```python
from build123d import *

# Parameters (mm, degrees)
SKETCH_1_R               = 51.220940725
EXTRUDE_1_DEPTH          = 2
SKETCH_2_R               = 3.5
EXTRUDE_2_DEPTH          = 5
PATTERN_CIRCULAR_1_COUNT = 6
SKETCH_3_R               = 2.5
CUT_EXTRUDE_1_DEPTH      = 3
PATTERN_CIRCULAR_2_COUNT = 6
SKETCH_4_R               = 2.5
EXTRUDE_3_DEPTH          = 11
SKETCH_5_R               = 3.5
EXTRUDE_4_DEPTH          = 7
SKETCH_6_R               = 5
EXTRUDE_5_DEPTH          = 20
SKETCH_7_R               = 6
EXTRUDE_6_DEPTH          = 5
SKETCH_8_R               = 2.5
CUT_EXTRUDE_2_DEPTH      = 7


with BuildPart() as part:
    # 草图1 → 凸台-拉伸1 (new body)
    with BuildSketch(Plane(origin=(0, 0, 0), x_dir=(0, 0, -1), z_dir=(1, 0, 0))):
        Circle(SKETCH_1_R)
    extrude(amount=EXTRUDE_1_DEPTH)

    # 草图2 → 凸台-拉伸2 (add)
    with BuildSketch(Plane(origin=(2, 0, 0), x_dir=(0, 0, -1), z_dir=(1, 0, 0))):
        with Locations((0, 45)):
            Circle(SKETCH_2_R)
    extrude_2 = extrude(amount=EXTRUDE_2_DEPTH)

    # 阵列(圆周)1: 凸台-拉伸2 ×6 about axis
    pattern_circular_1_axis = Axis((0, 0, 0), (1, 0, 0))
    for i in range(1, PATTERN_CIRCULAR_1_COUNT):
        add(extrude_2.rotate(pattern_circular_1_axis, i * 360 / PATTERN_CIRCULAR_1_COUNT))

    # 草图3 → 切除-拉伸1 (cut)
    with BuildSketch(Plane(origin=(7, 0, 0), x_dir=(0, 0, -1), z_dir=(1, 0, 0))):
        with Locations((0, 45)):
            Circle(SKETCH_3_R)
    cut_extrude_1 = extrude(amount=-CUT_EXTRUDE_1_DEPTH, mode=Mode.SUBTRACT)

    # 阵列(圆周)2: 切除-拉伸1 ×6 about axis
    pattern_circular_2_axis = Axis((0, 0, 0), (1, 0, 0))
    for i in range(1, PATTERN_CIRCULAR_2_COUNT):
        add(cut_extrude_1.rotate(pattern_circular_2_axis, i * 360 / PATTERN_CIRCULAR_2_COUNT), mode=Mode.SUBTRACT)

    # 草图4 → 凸台-拉伸3 (add)
    with BuildSketch(Plane(origin=(2, 0, 0), x_dir=(0, 0, -1), z_dir=(1, 0, 0))):
        Circle(SKETCH_4_R)
    extrude(amount=EXTRUDE_3_DEPTH)

    # 草图5 → 凸台-拉伸4 (add)
    with BuildSketch(Plane(origin=(2, 0, 0), x_dir=(0, 0, -1), z_dir=(1, 0, 0))):
        Circle(SKETCH_5_R)
    extrude(amount=EXTRUDE_4_DEPTH)

    # 草图6 → 凸台-拉伸5 (add)
    with BuildSketch(Plane.ZY):
        with Locations(Location((0, 0, 0), (0, 0, 180))):
            Circle(SKETCH_6_R)
    extrude(amount=EXTRUDE_5_DEPTH)

    # 草图7 → 凸台-拉伸6 (add)
    with BuildSketch(Plane.ZY):
        with Locations(Location((0, 0, 0), (0, 0, 180))):
            Circle(SKETCH_7_R)
    extrude(amount=EXTRUDE_6_DEPTH)

    # 草图8 → 切除-拉伸2 (cut)
    with BuildSketch(Plane.ZY.offset(20)):
        with Locations(Location((0, 0, 0), (0, 0, 180))):
            Circle(SKETCH_8_R)
    extrude(amount=-CUT_EXTRUDE_2_DEPTH, mode=Mode.SUBTRACT)


solid = part.part
```
For this review, take the finished solid that the model builds, in its own axes (mm). A direction names the side the tool comes from. Round coordinates to 2 decimals unless told otherwise and drop trailing zeros. Write each loop counter-clockwise with the first axis right and the second up, starting at its lowest first coordinate (ties: lowest second). Pieces come first, ordered by that corner, then holes. Notation, with made-up numbers: (48, -34) - (60, -34) arc R20 cw to (60, -17) - close; hole circle Ø4 at (1.5, 60.5). An arc over 180 degrees is marked (long way). Answer as CSV lines item,"result". Start each with the question number.
(1) Add section C-C, the plane z = 9. State the section outline as (x, y) points, plus the area to 3 significant figures.
(2) Add section D-D, the plane y = 45. State the section outline as (x, z) points, plus the area to 3 significant figures.
(3) Add section B-B, the plane x = 5.5. State how many separate pieces and enclosed holes the cut face has, plus the area to 3 significant figures.
(4) For pin 1 (1.5 mm diameter, centred on y = 23, z = -38, fed in from +X); pin 2 (5 mm diameter, centred on y = -34, z = 34, fed in from -X); pin 3 (8 mm diameter, centred on y = -22.5, z = 38.97, fed in from +X), all flat-tipped, find the tip position at first contact; note any pin that passes through.
(5) Machinability: for faces 5 (the flat face through (7, -23, -36)), 6 (the flat face through (4, -23, 39)), 7 (the cylindrical face through (-16.5, -0.1, 2.5)), which of the approach directions +Z, -Z, +X, -X, +Y, -Y give a long, thin tool a straight path to every point of the face, cutting with its end or side? Answer none if there is none.
(6) For line 1 (X direction, y = -17, z = -23.5); line 2 (X direction, y = 23.5, z = 37.5); line 3 (Y direction, x = 1.5, z = 19), list the stretches that pass through material, from the lowest coordinate up.
(7) Mouldability with a two-part tool opening along Y and no side actions: class faces 1 (the flat face through (-5, -4, 4)), 2 (the cylindrical face through (10.97, -2.44, 0.54)), 3 (the cylindrical face through (5.521, -22.39, -36.474)), 4 (the cylindrical face through (4.465, 20.135, -41.551)) as +Y half, -Y half, draft (parallel to the pull), parting line (faces both ways), or undercut.
(8) Add section A-A, the plane y = 0. State the section outline as (x, z) points, plus the area to 3 significant figures.
From the geometry:
1,outline,"(0, -50.42) - (2, -50.42) - (2, 50.42) - (0, 50.42) - close"
1,area,"202 mm²"
2,outline,"(0, -24.47) - (2, -24.47) - (2, -3.5) - (7, -3.5) - (7, -2.5) - (4, -2.5) - (4, 2.5) - (7, 2.5) - (7, 3.5) - (2, 3.5) - (2, 24.47) - (0, 24.47) - close"
2,area,"118 mm²"
3,separate pieces,"7"
3,enclosed holes,"6"
3,area,"152 mm²"
4,pin 1,"stops at x = 4"
4,pin 2,"stops at x = 0"
4,pin 3,"stops at x = 7"
5,face 5,"+Z, -Z, +X, +Y, -Y"
5,face 6,"+X"
5,face 7,"-X"
6,line 1,"x = 0 to 2"
6,line 2,"x = 0 to 4"
6,line 3,"y = -47.57 to 47.57"
7,face 1,"draft"
7,face 2,"parting line"
7,face 3,"undercut"
7,face 4,"undercut"
8,outline,"(-20, -5) - (-5, -5) - (-5, -6) - (0, -6) - (0, -51.22) - (2, -51.22) - (2, -3.5) - (9, -3.5) - (9, -2.5) - (13, -2.5) - (13, 2.5) - (9, 2.5) - (9, 3.5) - (2, 3.5) - (2, 51.22) - (0, 51.22) - (0, 6) - (-5, 6) - (-5, 5) - (-20, 5) - (-20, 2.5) - (-13, 2.5) - (-13, -2.5) - (-20, -2.5) - close"
8,area,"449 mm²"
